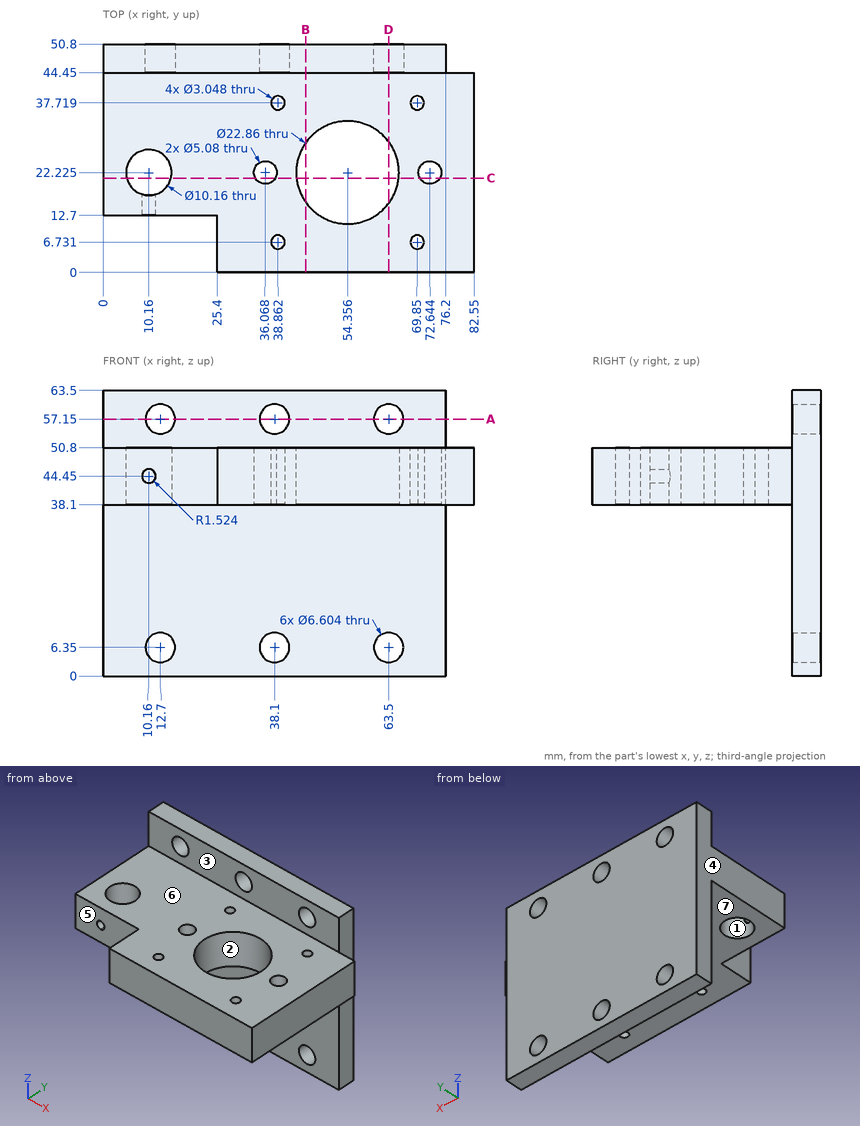
Check sheet for the drawn part. Datum: minimum x, y, z corner. Units: mm. A direction names the side the tool comes from. Round coordinates to 2 decimals unless told otherwise and drop trailing zeros. Order: outer loops, then holes, each group sorted by start corner. A loop starts at its lowest first (then second) coordinate and runs counter-clockwise, first axis right, second up. Notation, with made-up numbers: (66, 57.25) -> (73, 57.25) arc R11 ccw to (73, 69.25) -> close; hole circle Ø1 at (-37.5, 71.5). An arc over 180 degrees is marked (long way). Use CSV: the item, a comma, the result in double quotes.
(1) Tool access check on the marked faces 5, 6 and 7. Record the directions out of +Z, -Z, +X, -X, +Y, -Y that give a thin tool (end or side, any length) a straight path to the whole face; none if there is none.
Worked out:
face 5,"+Z, -Z, -X, -Y"
face 6,"+Z, +X, -X, -Y"
face 7,"-Z, +X, -X, -Y"
(2) Draft check along X on the marked faces 1, 2, 3 and 4. Enter one of: pulls with the +X half, pulls with the -X half, needs draft (parallel to the pull), parting line crosses it, or undercut.
Worked out:
face 1,"undercut"
face 2,"undercut"
face 3,"needs draft"
face 4,"pulls with the -X half"
(3) Depth check by flat-ended pin: pin 1 (14 mm diameter, centred on x = 11.5, z = 43, fed in from -Y); pin 2 (10.5 mm diameter, centred on x = 63.5, z = 57.15, fed in from -Y); pin 3 (3 mm diameter, centred on x = 80.5, z = 43, fed in from +Y). Enter the tip coordinate at first touch or a pass-through.
Worked out:
pin 1,"y = 12.7"
pin 2,"y = 44.45"
pin 3,"y = 44.45"
(4) Cross-section at A-A (z = 57.15). Record the boundary of the cut face in (x, y).
Worked out:
outline,"(0, 44.45) -> (9.4, 44.45) -> (9.4, 50.8) -> (0, 50.8) -> close; (16, 44.45) -> (34.8, 44.45) -> (34.8, 50.8) -> (16, 50.8) -> close; (41.4, 44.45) -> (60.2, 44.45) -> (60.2, 50.8) -> (41.4, 50.8) -> close; (66.8, 44.45) -> (76.2, 44.45) -> (76.2, 50.8) -> (66.8, 50.8) -> close"
(5) Cross-section at B-B (x = 45). Record the boundary of the cut face in (y, z).
Worked out:
outline,"(0, 38.1) -> (15.66, 38.1) -> (15.66, 50.8) -> (0, 50.8) -> close; (28.79, 38.1) -> (44.45, 38.1) -> (44.45, 0) -> (50.8, 0) -> (50.8, 63.5) -> (44.45, 63.5) -> (44.45, 50.8) -> (28.79, 50.8) -> close"
(6) Cross-section at C-C (y = 21). Record the boundary of the cut face in (x, z), and give its area (3 significant figures).
Worked out:
outline,"(0, 38.1) -> (5.23, 38.1) -> (5.23, 50.8) -> (0, 50.8) -> close; (15.09, 38.1) -> (33.84, 38.1) -> (33.84, 50.8) -> (15.09, 50.8) -> close; (38.29, 38.1) -> (42.99, 38.1) -> (42.99, 50.8) -> (38.29, 50.8) -> close; (65.72, 38.1) -> (70.42, 38.1) -> (70.42, 50.8) -> (65.72, 50.8) -> close; (74.87, 38.1) -> (82.55, 38.1) -> (82.55, 50.8) -> (74.87, 50.8) -> close"
area,"521 mm²"
(7) Cross-section at D-D (x = 63.5). Record the boundary of the cut face in (y, z).
Worked out:
outline,"(0, 38.1) -> (15.37, 38.1) -> (15.37, 50.8) -> (0, 50.8) -> close; (29.08, 38.1) -> (44.45, 38.1) -> (44.45, 9.65) -> (50.8, 9.65) -> (50.8, 53.85) -> (44.45, 53.85) -> (44.45, 50.8) -> (29.08, 50.8) -> close; (44.45, 0) -> (50.8, 0) -> (50.8, 3.05) -> (44.45, 3.05) -> close; (44.45, 60.45) -> (50.8, 60.45) -> (50.8, 63.5) -> (44.45, 63.5) -> close"
(8) Material ranges on line 1 along Y through (x, z) = (69.85, 45.5) (3 decimals); line 2 along Y through (x, z) = (70, 46); line 3 along X through (y, z) = (38, 48), recorded low to high. Write a range as from..to.
Worked out:
line 1,"0..5.207, 8.255..36.195, 39.243..50.8"
line 2,"0..5.21, 8.25..36.2, 39.24..50.8"
line 3,"0..37.36, 40.36..68.35, 71.35..82.55"
